```python
from build123d import *

# Parameters (mm, degrees)
SKETCH1_W           = 35.56
SKETCH1_H           = 35.56
BOSS_EXTRUDE1_DEPTH = 4.5
SKETCH2_W           = 35.56
SKETCH2_H           = 35.56
BOSS_EXTRUDE2_DEPTH = 2
SKETCH5_R           = 11
BOSS_EXTRUDE5_DEPTH = 2
SKETCH6_R           = 3.175
BOSS_EXTRUDE6_DEPTH = 24
SKETCH7_R           = 2
CUT_EXTRUDE3_DEPTH  = 29
SKETCH8_W           = 31.56
SKETCH8_H           = 31.56
BOSS_EXTRUDE7_DEPTH = 25
SKETCH9_W           = 35.56
SKETCH9_H           = 35.56
BOSS_EXTRUDE8_DEPTH = 6
CHAMFER1_SIZE       = 6


with BuildPart() as part:
    # Sketch1 → Boss-Extrude1 (new body)
    with BuildSketch(Plane.XY):
        with Locations((21.15, 20.624391857)):
            Rectangle(SKETCH1_W, SKETCH1_H)
    extrude(amount=BOSS_EXTRUDE1_DEPTH)

    # Sketch2 → Boss-Extrude2 (add)
    with BuildSketch(Plane.XY.offset(4.5)):
        with Locations((21.15, 20.624391857)):
            Rectangle(SKETCH2_W, SKETCH2_H)
    extrude(amount=BOSS_EXTRUDE2_DEPTH)

    # Sketch5 → Boss-Extrude5 (add)
    with BuildSketch(Plane(origin=(0, 0, 0), x_dir=(-1, 0, 0), z_dir=(0, 0, -1))):
        with Locations((-21.15, 20.624391857)):
            Circle(SKETCH5_R)
    extrude(amount=BOSS_EXTRUDE5_DEPTH)

    # Sketch6 → Boss-Extrude6 (add)
    with BuildSketch(Plane(origin=(0, 0, -2), x_dir=(-1, 0, 0), z_dir=(0, 0, -1))):
        with Locations((-21.15, 20.624391857)):
            Circle(SKETCH6_R)
    extrude(amount=BOSS_EXTRUDE6_DEPTH)

    # Sketch7 → Cut-Extrude3 (cut)
    with BuildSketch(Plane(origin=(0, 0, 0), x_dir=(-1, 0, 0), z_dir=(0, 0, -1))):
        with Locations((-35.65, 6.124391857)):
            Circle(SKETCH7_R)
        with Locations((-6.65, 6.124391857)):
            Circle(SKETCH7_R)
        with Locations((-6.65, 35.124391857)):
            Circle(SKETCH7_R)
        with Locations((-35.65, 35.124391857)):
            Circle(SKETCH7_R)
    extrude(amount=-CUT_EXTRUDE3_DEPTH, mode=Mode.SUBTRACT)

    # Sketch8 → Boss-Extrude7 (add)
    with BuildSketch(Plane.XY.offset(6.5)):
        with Locations((21.15, 20.624391857)):
            Rectangle(SKETCH8_W, SKETCH8_H)
    extrude(amount=BOSS_EXTRUDE7_DEPTH)

    # Sketch9 → Boss-Extrude8 (add)
    with BuildSketch(Plane.XY.offset(31.5)):
        with Locations((21.15, 20.624391857)):
            Rectangle(SKETCH9_W, SKETCH9_H)
    extrude(amount=BOSS_EXTRUDE8_DEPTH)

    # Chamfer1
    # the kernel refuses this chamfer: 6 mm, written as the material it takes off along each edge
    with BuildSketch(Plane(origin=(5.37, 36.404391857, 6.5), x_dir=(0.9996219169112968, 0.02749587661058678, 0), z_dir=(0, 0, 1)), Plane(origin=(36.93, 4.844391857, 6.5), x_dir=(-0.9996219169112969, -0.027495876610586355, 0), z_dir=(0, 0, 1)), Plane(origin=(36.93, 36.404391857, 6.5), x_dir=(0.02749587661058678, -0.9996219169112968, 0), z_dir=(0, 0, 1))) as chamfer1_piece_1:
        Polygon((CHAMFER1_SIZE * 0.999621916911, -CHAMFER1_SIZE * 0.0274958766106), (-CHAMFER1_SIZE * 0.0274958766106, -CHAMFER1_SIZE * 0.999621916911), (0, 0), align=None)
    extrude(amount=25, mode=Mode.SUBTRACT)
    with BuildSketch(Plane(origin=(5.37, 4.844391857, 6.5), x_dir=(0.9996219169112969, -0.027495876610586348, 0), z_dir=(0, 0, 1))) as chamfer1_piece_2:
        Polygon((CHAMFER1_SIZE * 0.999621916911, CHAMFER1_SIZE * 0.0274958766106), (-CHAMFER1_SIZE * 0.0274958766106, CHAMFER1_SIZE * 0.999621916911), (0, 0), align=None)
    extrude(amount=25, mode=Mode.SUBTRACT)


solid = part.part
```
Here's how the part is built. I have some questions about the finished solid (model axes, mm). A direction names the side the tool comes from. Round coordinates to 2 decimals unless told otherwise and drop trailing zeros. Loops run counter-clockwise (first coordinate to the right, second up) from the corner with the lowest first, then second, coordinate; pieces in that order, holes last. Notation, with made-up numbers: (54.5, 69) -> (73.5, 69) arc R14 ccw to (73.5, 86) -> close; hole circle Ø9 at (-27, 58.25). An arc over 180 degrees is marked (long way). Answer as CSV lines item,"result". Start each with the question number.
1. Imagine slicing it at C-C on y = 7. Write out the boundary of the cut face in (x, z), plus the area to 3 significant figures.
2. I need wall thicknesses on probe 1 along Y at (x, z) = (35.65, 2.75); probe 2 along Z at (x, y) = (5, 33.5); probe 3 along Z at (x, y) = (25.5, 32). Which ranges of each line are inside material? Lowest first, please. Write a range as from..to.
3. For faces 4 (the face through (5, 22, 31.5)), 5 (the face through (33.742, 6.725, 3.204)), 6 (the face through (8.412, 33.446, 18.825)), which set-ups out of +Z, -Z, +X, -X, +Y, -Y let a thin tool reach every point of the face, with its end or its side?
4. Imagine slicing it at B-B on z = 14. Write out the boundary of the cut face in (x, y), plus the area to 3 significant figures.
5. If we mould it in two halves opening along Y, with no side actions, what happens to faces 1 (the face through (29.257, 28.059, -0.986)), 2 (the face through (33.888, 7.802, 18.825)), 3 (the face through (6.91, 37.107, 3.204))? For each: pulls with the +Y half, pulls with the -Y half, needs draft (parallel to the pull), parting line crosses it, or undercut.
6. I'm going to push flat-ended pins straight in: P1, Ø6, axis at x = 11, y = 8.5, coming from the -Z side; P2, Ø2, axis at x = 22.5, z = 18, coming from the -Y side; P3, Ø3, axis at y = 18, z = -2, coming from the -X side. Where does each tip first touch, or does it pass through?
7. Imagine slicing it at D-D on x = 21.15. Write out the boundary of the cut face in (y, z).
8. Imagine slicing it at A-A on x = 35.5. Write out the boundary of the cut face in (y, z).
Solution:
1,outline,"(3.37, 0) -> (4.85, 0) -> (4.85, 6.5) -> (3.37, 6.5) -> close; (3.37, 31.5) -> (9.21, 31.5) -> (9.21, 6.5) -> (8.45, 6.5) -> (8.45, 0) -> (33.85, 0) -> (33.85, 6.5) -> (33.09, 6.5) -> (33.09, 31.5) -> (38.93, 31.5) -> (38.93, 37.5) -> (3.37, 37.5) -> close; (37.45, 0) -> (38.93, 0) -> (38.93, 6.5) -> (37.45, 6.5) -> close"
1,area,"995 mm²"
2,probe 1,"2.84..4.12, 8.12..33.12, 37.12..38.4"
2,probe 2,"0..6.5, 31.5..37.5"
2,probe 3,"0..37.5"
3,face 4,"none"
3,face 5,"-Z"
3,face 6,"-X, +Y"
4,outline,"(5.37, 10.84) -> (11.37, 4.84) -> (30.93, 4.84) -> (36.93, 10.84) -> (36.93, 30.4) -> (30.93, 36.4) -> (11.37, 36.4) -> (5.37, 30.4) -> close"
4,area,"924 mm²"
5,face 1,"parting line crosses it"
5,face 2,"pulls with the -Y half"
5,face 3,"undercut"
6,P1,"z = 0"
6,P2,"y = 4.84"
6,P3,"x = 10.21"
7,outline,"(2.84, 0) -> (9.62, 0) -> (9.62, -2) -> (17.45, -2) -> (17.45, -26) -> (23.8, -26) -> (23.8, -2) -> (31.62, -2) -> (31.62, 0) -> (38.4, 0) -> (38.4, 6.5) -> (36.4, 6.5) -> (36.4, 31.5) -> (38.4, 31.5) -> (38.4, 37.5) -> (2.84, 37.5) -> (2.84, 31.5) -> (4.84, 31.5) -> (4.84, 6.5) -> (2.84, 6.5) -> close"
8,outline,"(2.84, 0) -> (4.13, 0) -> (4.13, 6.5) -> (2.84, 6.5) -> close; (2.84, 31.5) -> (9.41, 31.5) -> (9.41, 6.5) -> (8.12, 6.5) -> (8.12, 0) -> (33.13, 0) -> (33.13, 6.5) -> (31.83, 6.5) -> (31.83, 31.5) -> (38.4, 31.5) -> (38.4, 37.5) -> (2.84, 37.5) -> close; (37.12, 0) -> (38.4, 0) -> (38.4, 6.5) -> (37.12, 6.5) -> close"
